Answer from the drawing. Dimensions are ordinates in mm from the lowest x, y and z of the part. Round coordinates to 2 decimals unless told otherwise and drop trailing zeros. Return JSON: item names as keys, results as strings. Group by question number.
(1) A cutting plane is placed at A-A on y = 57.15. State how many separate pieces and enclosed holes the cut face has, then the cut area to 3 significant figures.
(2) Given pin 1 (3 mm diameter, centred on x = 158.75, z = 50.8, fed in from -Y); pin 2 (10 mm diameter, centred on y = 8.5, z = 49.5, fed in from -X) (3 decimals); pin 3 (7.5 mm diameter, centred on x = 89, y = 11.5, fed in from -Z), each flat-ended and moving along its own axis, determine where each tip first touches the part or whether it passes through.
(3) Straight lines are drawn through the part: line 1 (Y direction, x = 91.5, z = 50.8) (1 decimal); line 2 (Z direction, x = 133.35, y = 35); line 3 (X direction, y = 46, z = 50.8). For each, find the intervals that lie inside material, in ascending order.
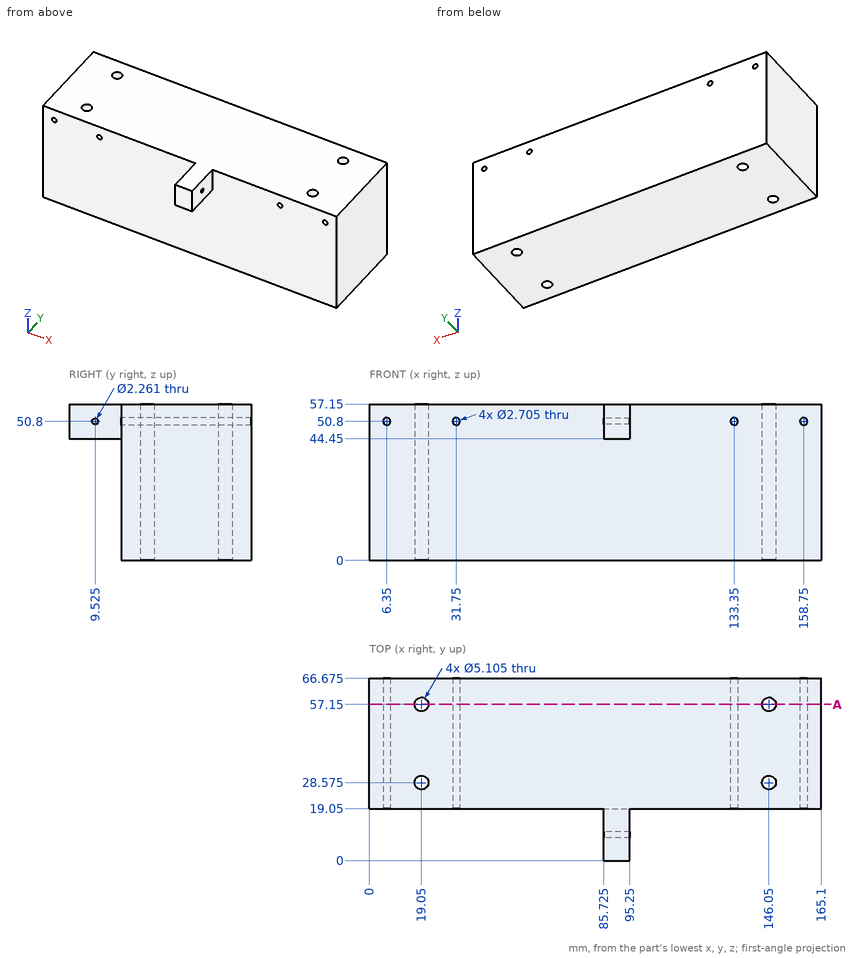
Checks:
{
 "1": {"separate pieces": "3", "enclosed holes": "4", "area": "8,830 mm^2"},
 "2": {"pin 1": "stops at y = 19.05", "pin 2": "stops at x = 85.725", "pin 3": "stops at z = 44.45"},
 "3": {"line 1": "y = 0 to 8.4, 10.7 to 66.7", "line 2": "z = 0 to 49.45, 52.15 to 57.15", "line 3": "x = 0 to 5, 7.7 to 30.4, 33.1 to 132, 134.7 to 157.4, 160.1 to 165.1"}
}
